For this review, take the finished solid that the model builds, in its own axes (mm). A direction names the side the tool comes from. Round coordinates to 2 decimals unless told otherwise and drop trailing zeros. Order: outer loops, then holes, each group sorted by start corner. A loop starts at its lowest first (then second) coordinate and runs counter-clockwise, first axis right, second up. Notation, with made-up numbers: (-35.75, 64.25) - (-9.75, 64.25) arc R13 cw to (-9.75, 80.25) - close; hole circle Ø8 at (21.25, -39.5). An arc over 180 degrees is marked (long way). One line per item, written item: value.
```python
from build123d import *

# Parameters (mm, degrees)
SKETCH1_W                                      = 38.1
SKETCH1_H                                      = 50.8
BOSS_EXTRUDE1_DEPTH                            = 6.35
CHAMFER1_SIZE                                  = 3.175
CBORE_FOR_6_SOCKET_HEAD_CAP_SCREW1_D           = 3.7973
CBORE_FOR_6_SOCKET_HEAD_CAP_SCREW1_CBORE_D     = 7.14502
CBORE_FOR_6_SOCKET_HEAD_CAP_SCREW1_CBORE_DEPTH = 4.191


with BuildPart() as part:
    # Sketch1 → Boss-Extrude1 (new body)
    with BuildSketch(Plane.XY):
        Rectangle(SKETCH1_W, SKETCH1_H)
    extrude(amount=-BOSS_EXTRUDE1_DEPTH)

    # Chamfer1
    chamfer1_edges = [part.edges().sort_by_distance(p)[0] for p in [
        (19.05, -25.4, -3.175),
        (-19.05, -25.4, -3.175),
        (-19.05, 25.4, -3.175),
        (19.05, 25.4, -3.175),
    ]]
    chamfer(chamfer1_edges, length=CHAMFER1_SIZE)

    # CBORE for #6 Socket Head Cap Screw1 (through all)
    with Locations(Plane(origin=(0, 0, -6.35), x_dir=(-1, 0, 0), z_dir=(0, 0, -1))):
        with Locations((0, -4.318), (0, 11.557)):
            CounterBoreHole(CBORE_FOR_6_SOCKET_HEAD_CAP_SCREW1_D / 2, CBORE_FOR_6_SOCKET_HEAD_CAP_SCREW1_CBORE_D / 2, CBORE_FOR_6_SOCKET_HEAD_CAP_SCREW1_CBORE_DEPTH)


solid = part.part
```
Item 1: Wall thickness on line 1 (Y direction, x = 0, z = -4.55); line 2 (Y direction, x = 0, z = -1.5); line 3 (Z direction, x = 0.5, y = -1.5): over which ranges is each line inside the solid? List them lowest first.
Returned:
line 1: -25.4 to -7.89, -0.75 to 7.98, 15.13 to 25.4
line 2: -25.4 to -6.22, -2.42 to 9.66, 13.46 to 25.4
line 3: -2.16 to 0
Item 2: Machinability: for faces 1 (the cylindrical face through (-0.41, -6.17, -1.06)), 2 (the cylindrical face through (0.465, -0.776, -4.284)), which of the approach directions +Z, -Z, +X, -X, +Y, -Y give a long, thin tool a straight path to every point of the face, cutting with its end or side? Answer none if there is none.
Returned:
face 1: +Z, -Z
face 2: -Z
Item 3: Take a section at B-B (z = -4.75). Count the separate pieces of the cut face and the enclosed holes in it, plus the area to 3 significant figures.
Returned:
separate pieces: 1
enclosed holes: 2
area: 1,840 mm^2
Item 4: Take a section at A-A (x = 0). Write out the cut boundary in (y, z).
Returned:
outline: (-25.4, -6.35) - (-7.89, -6.35) - (-7.89, -2.16) - (-6.22, -2.16) - (-6.22, 0) - (-25.4, 0) - close; (-2.42, -2.16) - (-0.75, -2.16) - (-0.75, -6.35) - (7.98, -6.35) - (7.98, -2.16) - (9.66, -2.16) - (9.66, 0) - (-2.42, 0) - close; (13.46, -2.16) - (15.13, -2.16) - (15.13, -6.35) - (25.4, -6.35) - (25.4, 0) - (13.46, 0) - close
Item 5: For P1, Ø3.5, axis at x = 1.5, y = -4, coming from the -Z side, flat-tipped, find the tip position at first contact; note if it passes through.
Returned:
P1: z = -2.16
Item 6: The part is to be moulded in two halves that separate along Y. For faces 3 (the cylindrical face through (0.77, 8.07, -4.28)), 4 (the cylindrical face through (-0.4, 9.7, -1.1)), 5 (the flat face through (-17.44, -23.835, -3.131)), 6 (the flat face through (-19.05, 0, -3)), say which applies: +Y half, -Y half, draft (parallel to the pull), parting line (faces both ways), or undercut.
Returned:
face 3: undercut
face 4: undercut
face 5: -Y half
face 6: draft
